Can you work these out from the model? Positions are in its coordinate system, mm. A direction names the side the tool comes from. Coordinates: 2 decimals unless noted, no trailing zeros. Order: outer loops, then holes, each group sorted by start corner. A loop starts at its lowest first (then second) coordinate and runs counter-clockwise, first axis right, second up. Notation, with made-up numbers: (-24, 55) -> (26, 55) arc R23 ccw to (26, 93) -> close; hole circle Ø11 at (55, 15.25). An arc over 180 degrees is marked (long way). Answer in a Markdown table with one row per item.
```python
from build123d import *

# Parameters (mm, degrees)
EXTRUDE_1_DEPTH          = 40
CUT_EXTRUDE_1_DEPTH      = 40
CUT_EXTRUDE_1_DEPTH_BACK = 40
SKETCH_2_W               = 4
SKETCH_2_H               = 12
SKETCH_3_R               = 1
EXTRUDE_2_DEPTH          = 10
EXTRUDE_START            = 10
SKETCH_4_R               = 1
EXTRUDE_3_DEPTH          = 10
CUT_EXTRUDE_2_DEPTH      = 10


with BuildPart() as part:
    # Sketch 1 → Extrude 1 (new body)
    with BuildSketch(Plane(origin=(0, 0, 0), x_dir=(1, 0, 0), z_dir=(0, 1, 0))):
        with BuildLine():
            ThreePointArc((-8, 1), (-8.585786438, -0.414213562), (-10, -1))
            Line((-10, -1), (10, -1))
            Line((10, -1), (10, 1))
            Line((10, 1), (-8, 1))
        make_face()
        with BuildLine():
            ThreePointArc((-8, 1), (-11.414213562, 2.414213562), (-10, -1))
            Line((-10, -1), (-10, 0))
            ThreePointArc((-10, 0), (-10.707106781, 1.707106781), (-9, 1))
            Line((-9, 1), (-8, 1))
        make_face()
        with BuildLine():
            Line((-10, 0), (-10, -1))
            ThreePointArc((-10, -1), (-8.585786438, -0.414213562), (-8, 1))
            Line((-8, 1), (-9, 1))
            ThreePointArc((-9, 1), (-9.292893219, 0.292893219), (-10, 0))
        make_face()
        with BuildLine():
            ThreePointArc((-9, 1), (-10.707106781, 1.707106781), (-10, 0))
            Line((-10, 0), (-10, 1))
            Line((-10, 1), (-9, 1))
        make_face()
        with BuildLine():
            Line((-10, 1), (-10, 0))
            ThreePointArc((-10, 0), (-9.292893219, 0.292893219), (-9, 1))
            Line((-9, 1), (-10, 1))
        make_face()
    extrude(amount=EXTRUDE_1_DEPTH)

    # Sketch 2 → Cut-Extrude 1 (cut, two sides: drawn at the far end of the back side and taken through both)
    with BuildSketch(Plane(origin=(0, 0, -1), x_dir=(-1, 0, 0), z_dir=(0, 0, -1)).offset(-CUT_EXTRUDE_1_DEPTH_BACK)):
        with Locations((10, 6)):
            Rectangle(SKETCH_2_W, SKETCH_2_H)
        with Locations((10, 34)):
            Rectangle(SKETCH_2_W, SKETCH_2_H)
    extrude(amount=CUT_EXTRUDE_1_DEPTH + CUT_EXTRUDE_1_DEPTH_BACK, mode=Mode.SUBTRACT)

    # Sketch 3 → Extrude 2 (add)
    with BuildSketch(Plane(origin=(0, 12, 0), x_dir=(-1, 0, 0), z_dir=(0, -1, 0))):
        with Locations(Location((10, 1, 0), (0, 0, 270))):
            Circle(SKETCH_3_R)
    extrude(amount=EXTRUDE_2_DEPTH)

    # Sketch 4 → Extrude 3 (add)
    with BuildSketch(Plane(origin=(0, 28, 0), x_dir=(1, 0, 0), z_dir=(0, 1, 0)).offset(EXTRUDE_START)):
        with Locations(Location((-10, 1, 0), (0, 0, 270))):
            Circle(SKETCH_4_R)
    extrude(amount=-EXTRUDE_3_DEPTH)

    # Sketch 5 → Cut-Extrude 2 (cut)
    with BuildSketch(Plane(origin=(0, 0, -1), x_dir=(-1, 0, 0), z_dir=(0, 0, -1))):
        with BuildLine():
            ThreePointArc((0.5, 32.5), (-0.378679656, 34.621320344), (-2.5, 35.5))
            Line((-2.5, 35.5), (-2.5, 32.5))
            Line((-2.5, 32.5), (-5.5, 32.5))
            ThreePointArc((-5.5, 32.5), (-2.5, 29.5), (0.5, 32.5))
        make_face()
        with BuildLine():
            Line((-2.5, 32.5), (-2.5, 35.5))
            ThreePointArc((-2.5, 35.5), (-4.621320344, 34.621320344), (-5.5, 32.5))
            Line((-5.5, 32.5), (-2.5, 32.5))
        make_face()
        with BuildLine():
            ThreePointArc((-5.5, 7.5), (-4.621320344, 5.378679656), (-2.5, 4.5))
            Line((-2.5, 4.5), (-2.5, 7.5))
            Line((-2.5, 7.5), (-5.5, 7.5))
        make_face()
        with BuildLine():
            Line((-2.5, 7.5), (-2.5, 4.5))
            ThreePointArc((-2.5, 4.5), (-0.378679656, 5.378679656), (0.5, 7.5))
            ThreePointArc((0.5, 7.5), (-2.5, 10.5), (-5.5, 7.5))
            Line((-5.5, 7.5), (-2.5, 7.5))
        make_face()
    extrude(amount=-CUT_EXTRUDE_2_DEPTH, mode=Mode.SUBTRACT)


solid = part.part
```
(1) We'd pull the mould along X, two halves only. Please class faces 6 (the cylindrical face through (-11.367, 19.888, -2.46)), 7 (the cylindrical face through (-9, 33, -1)), 8 (the flat face through (1, 0, 0)): +X half, -X half, draft (parallel to the pull), parting line (faces both ways), or undercut.
Response values:
| item | result |
|---|---|
| face 6 | parting line |
| face 7 | undercut |
| face 8 | draft |
(2) Will these pins go through, and if not, where does the flat tip stop? pin 1 Ø2 at (x, z) = (-10, -1) entering from -Y; pin 2 Ø1.2 at (x, z) = (-10, -1) entering from +Y; pin 3 Ø1.6 at (y, z) = (33.5, 0) entering from -X; pin 4 Ø1.5 at (x, z) = (1.5, -2.5) entering from +Y.
Response values:
| item | result |
|---|---|
| pin 1 | y = 2 |
| pin 2 | y = 38 |
| pin 3 | x = -10.98 |
| pin 4 | through |
(3) Suppose I cut it at D-D (y = 24.5). Please give me the cut outline in (x, z), and give its area (3 significant figures).
Response values:
| item | result |
|---|---|
| outline | (-10, 1) arc R2 ccw (long way) to (-8, -1) -> (10, -1) -> (10, 1) -> close |
| area | 49.4 mm2 |
(4) Suppose I cut it at A-A (y = 29). Please give me the cut outline in (x, z), and give its area (3 significant figures).
Response values:
| item | result |
|---|---|
| outline | circle Ø2 at (-10, -1); (-8, -1) -> (10, -1) -> (10, 1) -> (-8, 1) -> close |
| area | 39.1 mm2 |
(5) Suppose I cut it at B-B (z = -0.6). Please give me the cut outline in (x, y).
Response values:
| item | result |
|---|---|
| outline | (-11.96, 12) -> (-10.92, 12) -> (-10.92, 2) -> (-9.08, 2) -> (-9.08, 12) -> (-8, 12) -> (-8, 0) -> (10, 0) -> (10, 40) -> (-8, 40) -> (-8, 28) -> (-9.08, 28) -> (-9.08, 38) -> (-10.92, 38) -> (-10.92, 28) -> (-11.96, 28) -> close; hole circle Ø6 at (2.5, 7.5); hole circle Ø6 at (2.5, 32.5) |
(6) On a 3-axis mill with a long thin cutter (end or side, diameter ignored), from which of +Z, -Z, +X, -X, +Y, -Y can I reach the whole of each face in a straight line? I mean faces 1 (the flat face through (-8, 34, 0)), 2 (the cylindrical face through (-11, 7, -1)), 3 (the flat face through (-10, 38, -1)), 4 (the flat face through (-10, 2, -1)), 5 (the flat face through (-9, 28, 0)). Say none if no direction works.
Response values:
| item | result |
|---|---|
| face 1 | +Z, -Z, +Y |
| face 2 | -Y |
| face 3 | +Z, -Z, -X, +Y |
| face 4 | +Z, -Z, -X, -Y |
| face 5 | +Y |
(7) Suppose I cut it at C-C (x = 6.75). Please give me the cut outline in (y, z).
Response values:
| item | result |
|---|---|
| outline | (0, -1) -> (40, -1) -> (40, 1) -> (0, 1) -> close |
(8) I need wall thicknesses on line 1 (Y direction, x = 1, z = -0.5); line 2 (X direction, y = 33, z = -0.85); line 3 (Z direction, x = -2.25, y = 13). Which ranges of each line are inside material? Lowest first, please. Write a range as [from, to].
Response values:
| item | result |
|---|---|
| line 1 | [0, 4.9], [10.1, 29.9], [35.1, 40] |
| line 2 | [-10.99, -9.01], [-8, -0.46], [5.46, 10] |
| line 3 | [-1, 1] |
